Model file for the job. Use its own axes, mm. Face numbers are marked on the shaded views. A direction names the side the tool comes from. Coordinates: 2 decimals unless noted, no trailing zeros. Loops run counter-clockwise (first coordinate to the right, second up) from the corner with the lowest first, then second, coordinate; pieces in that order, holes last. Notation, with made-up numbers: (47, 53.25) -> (57, 53.25) arc R20 cw to (57, 72.25) -> close; hole circle Ø5 at (52.25, 70). An arc over 180 degrees is marked (long way). Use one line per item in the form item = value.
```python
from build123d import *

# Parameters (mm, degrees)
EXTRUDE_1_DEPTH     = 2
EXTRUDE_START       = 20
EXTRUDE_3_DEPTH     = 20
SKETCH_1_5_R        = 2.5
SKETCH_1_5_R_2      = 1.45
EXTRUDE_4_DEPTH     = 2
CUT_EXTRUDE_2_DEPTH = 2
CUT_EXTRUDE_3_DEPTH = 2


with BuildPart() as part:
    # Sketch 1 → Extrude 1 (new body)
    with BuildSketch(Plane(origin=(0, 0, 0), x_dir=(1, 0, 0), z_dir=(0, 1, 0))):
        with BuildLine():
            Line((-40, 24), (40, 24))
            ThreePointArc((40, 24), (41.414213562, 23.414213562), (42, 22))
            Line((42, 22), (42, -22))
            ThreePointArc((42, -22), (41.414213562, -23.414213562), (40, -24))
            Line((40, -24), (-40, -24))
            ThreePointArc((-40, -24), (-41.414213562, -23.414213562), (-42, -22))
            Line((-42, -22), (-42, 22))
            ThreePointArc((-42, 22), (-41.414213562, 23.414213562), (-40, 24))
        make_face()
    extrude(amount=-EXTRUDE_1_DEPTH)

    # Sketch 1_4 → Extrude 3 (add)
    with BuildSketch(Plane(origin=(0, 0, 0), x_dir=(1, 0, 0), z_dir=(0, 1, 0)).offset(EXTRUDE_START)):
        with BuildLine():
            Line((-40, 24), (40, 24))
            ThreePointArc((40, 24), (41.414213562, 23.414213562), (42, 22))
            Line((42, 22), (42, -22))
            ThreePointArc((42, -22), (41.414213562, -23.414213562), (40, -24))
            Line((40, -24), (-40, -24))
            ThreePointArc((-40, -24), (-41.414213562, -23.414213562), (-42, -22))
            Line((-42, -22), (-42, 22))
            ThreePointArc((-42, 22), (-41.414213562, 23.414213562), (-40, 24))
        make_face()
        with BuildLine():
            Line((-38, 22), (38, 22))
            ThreePointArc((38, 22), (39.414213562, 21.414213562), (40, 20))
            Line((40, 20), (40, -20))
            ThreePointArc((40, -20), (39.414213562, -21.414213562), (38, -22))
            Line((38, -22), (-38, -22))
            ThreePointArc((-38, -22), (-39.414213562, -21.414213562), (-40, -20))
            Line((-40, -20), (-40, 20))
            ThreePointArc((-40, 20), (-39.414213562, 21.414213562), (-38, 22))
        make_face(mode=Mode.SUBTRACT)
    extrude(amount=-EXTRUDE_3_DEPTH)

    # Sketch 1_5 → Extrude 4 (add)
    # profile 1 of 4: a face of its own
    with BuildSketch(Plane(origin=(0, 0, 0), x_dir=(1, 0, 0), z_dir=(0, 1, 0))):
        with Locations(Location((-35, 17.5, 0), (0, 0, 90))):
            Circle(SKETCH_1_5_R)
        with Locations(Location((-35, 17.5, 0), (0, 0, 270))):
            Circle(SKETCH_1_5_R_2, mode=Mode.SUBTRACT)
    # profile 2 of 4: a face of its own
    with BuildSketch(Plane(origin=(0, 0, 0), x_dir=(1, 0, 0), z_dir=(0, 1, 0))):
        with Locations(Location((35, 17.5, 0), (0, 0, 90))):
            Circle(SKETCH_1_5_R)
        with Locations(Location((35, 17.5, 0), (0, 0, 270))):
            Circle(SKETCH_1_5_R_2, mode=Mode.SUBTRACT)
    # profile 3 of 4: a face of its own
    with BuildSketch(Plane(origin=(0, 0, 0), x_dir=(1, 0, 0), z_dir=(0, 1, 0))):
        with Locations(Location((35, -17.5, 0), (0, 0, 90))):
            Circle(SKETCH_1_5_R)
        with Locations(Location((35, -17.5, 0), (0, 0, 270))):
            Circle(SKETCH_1_5_R_2, mode=Mode.SUBTRACT)
    # profile 4 of 4: a face of its own
    with BuildSketch(Plane(origin=(0, 0, 0), x_dir=(1, 0, 0), z_dir=(0, 1, 0))):
        with Locations(Location((-35, -17.5, 0), (0, 0, 90))):
            Circle(SKETCH_1_5_R)
        with Locations(Location((-35, -17.5, 0), (0, 0, 270))):
            Circle(SKETCH_1_5_R_2, mode=Mode.SUBTRACT)
    extrude(amount=EXTRUDE_4_DEPTH)

    # Sketch 2 → Cut-Extrude 2 (cut)
    with BuildSketch(Plane.XZ.offset(2)):
        Polygon((30, 5.185127278), (26, -17.5), (30, -17.5), align=None)
        Polygon((28.171444325, 17.5), (24.171444325, 17.5), (18, -17.5), (22, -17.5), align=None)
        Polygon((20.171444325, 17.5), (16.171444325, 17.5), (10, -17.5), (14, -17.5), align=None)
        Polygon((12.171444325, 17.5), (8.171444325, 17.5), (2, -17.5), (6, -17.5), align=None)
        Polygon((4.171444325, 17.5), (0.171444325, 17.5), (-6, -17.5), (-2, -17.5), align=None)
        Polygon((-3.828555675, 17.5), (-7.828555675, 17.5), (-14, -17.5), (-10, -17.5), align=None)
        Polygon((-11.828555675, 17.5), (-15.828555675, 17.5), (-22, -17.5), (-18, -17.5), align=None)
        Polygon((-19.828555675, 17.5), (-23.828555675, 17.5), (-30, -17.5), (-26, -17.5), align=None)
        Polygon((-30, 5.185127278), (-27.828555675, 17.5), (-30, 17.5), align=None)
    extrude(amount=-CUT_EXTRUDE_2_DEPTH, mode=Mode.SUBTRACT)

    # Sketch 3 → Cut-Extrude 3 (cut)
    with BuildSketch(Plane(origin=(-40, 0, 0), x_dir=(0, 0, -1), z_dir=(1, 0, 0))):
        with BuildLine():
            Line((-10.25, 6), (-10.25, 12))
            ThreePointArc((-10.25, 12), (-9.664213562, 13.414213562), (-8.25, 14))
            Line((-8.25, 14), (8.25, 14))
            ThreePointArc((8.25, 14), (9.664213562, 13.414213562), (10.25, 12))
            Line((10.25, 12), (10.25, 6))
            ThreePointArc((10.25, 6), (9.664213562, 4.585786438), (8.25, 4))
            Line((8.25, 4), (-8.25, 4))
            ThreePointArc((-8.25, 4), (-9.664213562, 4.585786438), (-10.25, 6))
        make_face()
    extrude(amount=-CUT_EXTRUDE_3_DEPTH, mode=Mode.SUBTRACT)


solid = part.part
```
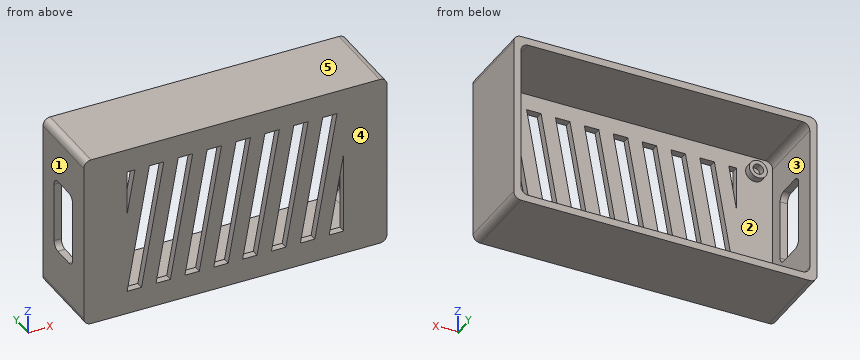
Q1. Wall check: line 1 along X through (y, z) = (0.55, -17.5); line 2 along Z through (x, y) = (-28, 11); line 3 along X through (y, z) = (17.75, 1.5). Give the ranges that are in metal, low to high.
Result:
line_1 = -42 to -40, -37.5 to -36.45, -33.55 to -32.5, 32.5 to 33.55, 36.45 to 37.5, 40 to 42
line_2 = -24 to -22, 22 to 24
line_3 = -42 to -40, 40 to 42
Q2. Band-saw the part on D-D, the plane z = 7. State how many separate pieces and enclosed holes the cut face has, and give its area (3 significant figures).
Result:
separate_pieces = 10
enclosed_holes = 0
area = 171 mm2
Q3. Mould opens along Z. For the marked faces 3, 4 and 5 say: released by +Z, released by -Z, zero draft, split by the parting line, or undercut.
Result:
face_3 = undercut
face_4 = zero draft
face_5 = released by +Z
Q4. Which spindle directions (+Z, -Z, +X, -X, +Y, -Y) get a long thin tool onto all of the face, cutting with end or side? Do the marked faces 1 and 2. Say none if no direction does.
Result:
face_1 = +Z, -Z, -X, +Y, -Y
face_2 = +Y
Q5. Pin check, flat tips, straight feed: pin 1 Ø4 at (x, z) = (34, 17) entering from +Y; pin 2 Ø1 at (x, z) = (30, 14.5) entering from +Y. Stop position of each tip, or through.
Result:
pin_1 = 2
pin_2 = 0
Q6. Band-saw the part on C-C, the plane y = 18.5. Write the cut outline in (x, z), and give its area (3 significant figures).
Result:
outline = (-42, -22) arc R2 ccw to (-40, -24) -> (40, -24) arc R2 ccw to (42, -22) -> (42, 22) arc R2 ccw to (40, 24) -> (-40, 24) arc R2 ccw to (-42, 22) -> close; hole (-40, -20) arc R2 ccw to (-38, -22) -> (38, -22) arc R2 ccw to (40, -20) -> (40, 20) arc R2 ccw to (38, 22) -> (-38, 22) arc R2 ccw to (-40, 20) -> close
area = 512 mm2
Q7. Band-saw the part on B-B, the plane y = 7. Write the cut outline in (x, z), and give its area (3 significant figures).
Result:
outline = (-42, -22) arc R2 ccw to (-40, -24) -> (40, -24) arc R2 ccw to (42, -22) -> (42, 22) arc R2 ccw to (40, 24) -> (-40, 24) arc R2 ccw to (-42, 22) -> (-42, 10.25) -> (-40, 10.25) -> (-40, 20) arc R2 cw to (-38, 22) -> (38, 22) arc R2 cw to (40, 20) -> (40, -20) arc R2 cw to (38, -22) -> (-38, -22) arc R2 cw to (-40, -20) -> (-40, -10.25) -> (-42, -10.25) -> close
area = 471 mm2
Q8. Band-saw the part on A-A, the plane x = -35. Write the cut outline in (y, z), and give its area (3 significant figures).
Result:
outline = (-2, -24) -> (20, -24) -> (20, -22) -> (0, -22) -> (0, -20) -> (2, -20) -> (2, -18.95) -> (0, -18.95) -> (0, -16.05) -> (2, -16.05) -> (2, -15) -> (0, -15) -> (0, 15) -> (2, 15) -> (2, 16.05) -> (0, 16.05) -> (0, 18.95) -> (2, 18.95) -> (2, 20) -> (0, 20) -> (0, 22) -> (20, 22) -> (20, 24) -> (-2, 24) -> close
area = 184 mm2
